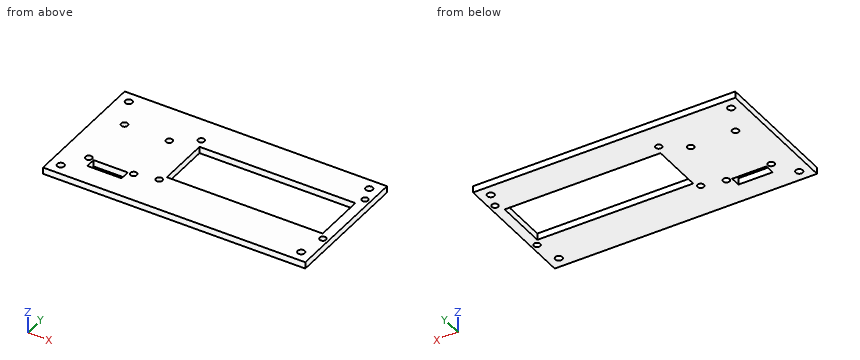
```python
from build123d import *

# Parameters (mm, degrees)
SKETCH1_W           = 120
SKETCH1_H           = 60
BOSS_EXTRUDE1_DEPTH = 3
SKETCH3_R           = 1.6
CUT_EXTRUDE2_DEPTH  = 73.520148402
SKETCH5_R           = 1.45
CUT_EXTRUDE4_DEPTH  = 73.520148402
SKETCH7_W           = 71.3
SKETCH7_H           = 24
CUT_EXTRUDE5_DEPTH  = 73.520148402
SKETCH8_R           = 1.5
SKETCH8_W           = 15.689778119
SKETCH8_H           = 4.586192705
CUT_EXTRUDE6_DEPTH  = 73.520148402


with BuildPart() as part:
    # Sketch1 → Boss-Extrude1 (new body)
    with BuildSketch(Plane.XY):
        with Locations((3.092575742, -5.63002681)):
            Rectangle(SKETCH1_W, SKETCH1_H)
    extrude(amount=BOSS_EXTRUDE1_DEPTH)

    # Sketch3 → Cut-Extrude2 (cut, through all)
    with BuildSketch(Plane.XY.offset(3)):
        with Locations((58.092575742, 19.36997319)):
            Circle(SKETCH3_R)
        with Locations((58.092575742, -30.63002681)):
            Circle(SKETCH3_R)
        with Locations((-51.907424258, -30.63002681)):
            Circle(SKETCH3_R)
        with Locations((-51.907424258, 19.36997319)):
            Circle(SKETCH3_R)
    extrude(amount=-CUT_EXTRUDE2_DEPTH, mode=Mode.SUBTRACT)

    # Sketch5 → Cut-Extrude4 (cut, through all)
    with BuildSketch(Plane(origin=(0, 0, 0), x_dir=(-1, 0, 0), z_dir=(0, 0, -1))):
        with Locations((14.357424258, 12.31997319)):
            Circle(SKETCH5_R)
        with Locations((14.357424258, -18.58002681)):
            Circle(SKETCH5_R)
        with Locations((-60.542575742, -18.58002681)):
            Circle(SKETCH5_R)
        with Locations((-60.542575742, 12.31997319)):
            Circle(SKETCH5_R)
    extrude(amount=-CUT_EXTRUDE4_DEPTH, mode=Mode.SUBTRACT)

    # Sketch7 → Cut-Extrude5 (cut, through all)
    with BuildSketch(Plane.XY.offset(3)):
        with Locations((22.992575742, -3.73002681)):
            Rectangle(SKETCH7_W, SKETCH7_H)
    extrude(amount=-CUT_EXTRUDE5_DEPTH, mode=Mode.SUBTRACT)

    # Sketch8 → Cut-Extrude6 (cut, through all)
    with BuildSketch(Plane.XY.offset(3)):
        with Locations((-45.257424258, 5.51997319)):
            Circle(SKETCH8_R)
        with Locations((-24.757424258, 5.51997319)):
            Circle(SKETCH8_R)
        with Locations((-24.757424258, -20.68002681)):
            Circle(SKETCH8_R)
        with Locations((-45.257424258, -20.68002681)):
            Circle(SKETCH8_R)
        with Locations((-35.029761386, -23.336930458)):
            Rectangle(SKETCH8_W, SKETCH8_H)
    extrude(amount=-CUT_EXTRUDE6_DEPTH, mode=Mode.SUBTRACT)


solid = part.part
```
Here's how the part is built. I have some questions about the finished solid (model axes, mm). Round coordinates to 2 decimals unless told otherwise and drop trailing zeros. Order: outer loops, then holes, each group sorted by start corner. A loop starts at its lowest first (then second) coordinate and runs counter-clockwise, first axis right, second up. Notation, with made-up numbers: (87.25, 49) -> (114.25, 49) arc R23 ccw to (114.25, 79) -> close; hole circle Ø1 at (40.25, 84). An arc over 180 degrees is marked (long way). Use a Markdown table: item, result. Add a question column.
(1) Suppose I cut it at C-C, the plane z = 1. Count the separate pieces of the cut face and the enclosed holes in it, and give its area (3 significant figures).
(2) I need wall thicknesses on line 1 along Y through (x, z) = (-14.5, 2.75); line 2 along X through (y, z) = (-12, 1.1); line 3 along Y through (x, z) = (-23.5, 2.25). Which ranges of each line are inside material? Lowest first, please.
(3) Suppose I cut it at A-A, the plane x = 4. Please give me the cut outline in (y, z).
(4) Suppose I cut it at B-B, the plane y = -2.5. Please give me the cut outline in (x, z).
Verdict:
| question | item | result |
|---|---|---|
| 1 | separate pieces | 1 |
| 1 | enclosed holes | 14 |
| 1 | area | 5,330 mm2 |
| 2 | line 1 | -35.63 to -20.02, -17.14 to 10.88, 13.76 to 24.37 |
| 2 | line 2 | -56.91 to -12.66, 58.64 to 63.09 |
| 2 | line 3 | -35.63 to -21.5, -19.86 to 4.7, 6.34 to 24.37 |
| 3 | outline | (-35.63, 0) -> (-15.73, 0) -> (-15.73, 3) -> (-35.63, 3) -> close; (8.27, 0) -> (24.37, 0) -> (24.37, 3) -> (8.27, 3) -> close |
| 4 | outline | (-56.91, 0) -> (-12.66, 0) -> (-12.66, 3) -> (-56.91, 3) -> close; (58.64, 0) -> (63.09, 0) -> (63.09, 3) -> (58.64, 3) -> close |
